from build123d import *

# Parameters (mm, degrees)
F0_W     = 6.9
F0_H     = 11.77
F1_DEPTH = 2
F2_DEPTH = 11
F3_R     = 0.5


with BuildPart() as f1:
    # F0 (on Top) → F1 (new body)
    with BuildSketch(Plane.XY):
        Polygon((-2.3468033714, 10.8328205479), (-5.95, 6.8476179095), (-5.95, -8.385), (5.95, -8.385), (5.95, 6.8476179095), (2.3468033714, 10.8328205479), align=None)
        Polygon((-4.95, -7.385), (-4.95, 6.4625707457), (-1.9028092228, 9.8328205479), (1.9028092228, 9.8328205479), (4.95, 6.4625707457), (4.95, -7.385), align=None, mode=Mode.SUBTRACT)
        Polygon((-1.9028092228, 9.8328205479), (-4.95, 6.4625707457), (-4.95, -7.385), (4.95, -7.385), (4.95, 6.4625707457), (1.9028092228, 9.8328205479), align=None)
        Polygon((1.236818, 8.3328205479), (3.45, 5.885), (3.45, -5.885), (-3.45, -5.885), (-3.45, 5.885), (-1.236818, 8.3328205479), align=None, mode=Mode.SUBTRACT)
        Polygon((-3.45, 5.885), (3.45, 5.885), (1.236818, 8.3328205479), (-1.236818, 8.3328205479), align=None)
        Rectangle(F0_W, F0_H)
    extrude(amount=F1_DEPTH)

    # F0 (on Top) → F2 (join)
    with BuildSketch(Plane.XY):
        Polygon((-1.9028092228, 9.8328205479), (-4.95, 6.4625707457), (-4.95, -7.385), (4.95, -7.385), (4.95, 6.4625707457), (1.9028092228, 9.8328205479), align=None)
        Polygon((1.236818, 8.3328205479), (3.45, 5.885), (3.45, -5.885), (-3.45, -5.885), (-3.45, 5.885), (-1.236818, 8.3328205479), align=None, mode=Mode.SUBTRACT)
    extrude(amount=F2_DEPTH)

    # F3
    f3_edges = [f1.edges().sort_by_distance(p)[0] for p in [
        (-3.45, 0, 2),
        (-2.343409, 7.10891, 2),
        (0, 8.332821, 2),
        (2.343409, 7.10891, 2),
        (3.45, 0, 2),
        (0, -5.885, 2),
        (0, -7.385, 2),
        (4.95, -0.461215, 2),
        (3.426405, 8.147696, 2),
        (0, 9.832821, 2),
        (-3.426405, 8.147696, 2),
        (-4.95, -0.461215, 2),
    ]]
    fillet(f3_edges, radius=F3_R)


solid = f1.part
Check sheet for the modelled part. Datum: model origin and axes. Units: mm. A direction names the side the tool comes from. Round coordinates to 2 decimals unless told otherwise and drop trailing zeros. Order: outer loops, then holes, each group sorted by start corner. A loop starts at its lowest first (then second) coordinate and runs counter-clockwise, first axis right, second up.
(1) Cross-section at D-D, the plane y = 5. Enter the section's corners in (x, z).
(2) Access from +Z, -Z, +X, -X, +Y, -Y to the whole of each face (thin tool, end or side, straight path). Record for faces 1 (the flat face through (-4.95, 0, 7)), 2 (the flat face through (0, 9.833, 7)), 3 (the flat face through (0, 1, 2)), 4 (the flat face through (0, -7.385, 7)), 5 (the flat face through (-3.405, 8.171, 6.69)).
(3) Draft check along Y on faces 6 (the flat face through (-4, 1, 11)), 7 (the flat face through (-4.12, 8.87, 0.99)), 8 (the cylindrical face through (2.22, 7.03, 2.15)), 9 (the flat face through (3.45, 0, 7)). Enter one of: pulls with the +Y half, pulls with the -Y half, needs draft (parallel to the pull), parting line crosses it, or undercut.
(4) Cross-section at B-B, the plane y = -7. Enter the section's corners in (x, z), and give its area (3 significant figures).
(5) Cross-section at C-C, the plane x = 0.5. Enter the section's corners in (y, z) (3 decimals), and give its area (3 significant figures).
(6) Go/stop test with flat-tipped pins: P1, Ø2, axis at x = 0.5, z = 6.5, coming from the +Y side; P2, Ø0.7, axis at x = -0.5, z = 6, coming from the -Y side (3 decimals); P3, Ø6.5, axis at x = 0, y = -1, coming from the +Z side. Record where each tip stops, or that it passes through.
(7) Scan lines: probe 1 along X at (y, z) = (0.25, 9.5); probe 2 along Z at (x, y) = (0.5, 0). Record each from-to range of solid material in increasing order.
(8) Cross-section at A-A, the plane z = 5.25. Enter the section's corners in (x, y) (3 decimals), and give its area (3 significant figures).
Check sheet entries:
1. outline: (-5.95, 0) - (5.95, 0) - (5.95, 2) - (5.45, 2) arc R0.5 cw to (4.95, 2.5) - (4.95, 11) - (3.45, 11) - (3.45, 2.5) arc R0.5 cw to (2.95, 2) - (-2.95, 2) arc R0.5 cw to (-3.45, 2.5) - (-3.45, 11) - (-4.95, 11) - (-4.95, 2.5) arc R0.5 cw to (-5.45, 2) - (-5.95, 2) - close
2. face 1: +Z, -X, +Y, -Y
2. face 2: +Z, +X, -X, +Y
2. face 3: +Z
2. face 4: +Z, +X, -X, -Y
2. face 5: +Z, -X, +Y
3. face 6: needs draft
3. face 7: pulls with the +Y half
3. face 8: undercut
3. face 9: undercut
4. outline: (-5.95, 0) - (5.95, 0) - (5.95, 2) - (5.45, 2) arc R0.5 cw to (4.95, 2.5) - (4.95, 11) - (-4.95, 11) - (-4.95, 2.5) arc R0.5 cw to (-5.45, 2) - (-5.95, 2) - close
4. area: 113 mm2
5. outline: (-8.385, 0) - (10.833, 0) - (10.833, 2) - (10.333, 2) arc R0.5 cw to (9.833, 2.5) - (9.833, 11) - (8.333, 11) - (8.333, 2.5) arc R0.5 cw to (7.833, 2) - (-5.385, 2) arc R0.5 cw to (-5.885, 2.5) - (-5.885, 11) - (-7.385, 11) - (-7.385, 2.5) arc R0.5 cw to (-7.885, 2) - (-8.385, 2) - close
5. area: 65.7 mm2
6. P1: stops at y = 9.83
6. P2: stops at y = -7.385
6. P3: stops at z = 2.1
7. probe 1: x = -4.95 to -3.45, 3.45 to 4.95
7. probe 2: z = 0 to 2
8. outline: (-4.95, -7.385) - (4.95, -7.385) - (4.95, 6.463) - (1.903, 9.833) - (-1.903, 9.833) - (-4.95, 6.463) - close; hole (-3.45, -5.885) - (3.45, -5.885) - (3.45, 5.885) - (1.237, 8.333) - (-1.237, 8.333) - (-3.45, 5.885) - close
8. area: 67.5 mm2
